For this review, use the dimensioned drawing (mm, ordinates from the lowest corner) and the shaded views. Coordinates: 2 decimals unless noted, no trailing zeros. Loops run counter-clockwise (first coordinate to the right, second up) from the corner with the lowest first, then second, coordinate; pieces in that order, holes last.
1. Take a section at A-A, the plane x = 105. State the section outline as (y, z) points.
2. Take a section at C-C, the plane y = 4.5. State the section outline as (x, z) points.
3. Clearance check with a flat-ended pin moving along its axis: P1, Ø14.5, axis at x = 283, z = 11, coming from the -Y side. State where the tip first meets the part, or that it passes through.
4. To check wall thickness, follow probe 1 along X at (y, z) = (6, 283); probe 2 along X at (y, z) = (5.5, 28); probe 3 along Z at (x, y) = (216, 1.5). State the ranges of each line that lie inside material, in increasing order.
5. Take a section at B-B, the plane z = 220.5. State the section outline as (x, y) points.
6. Take a section at D-D, the plane z = 283. State the section outline as (x, y) points.
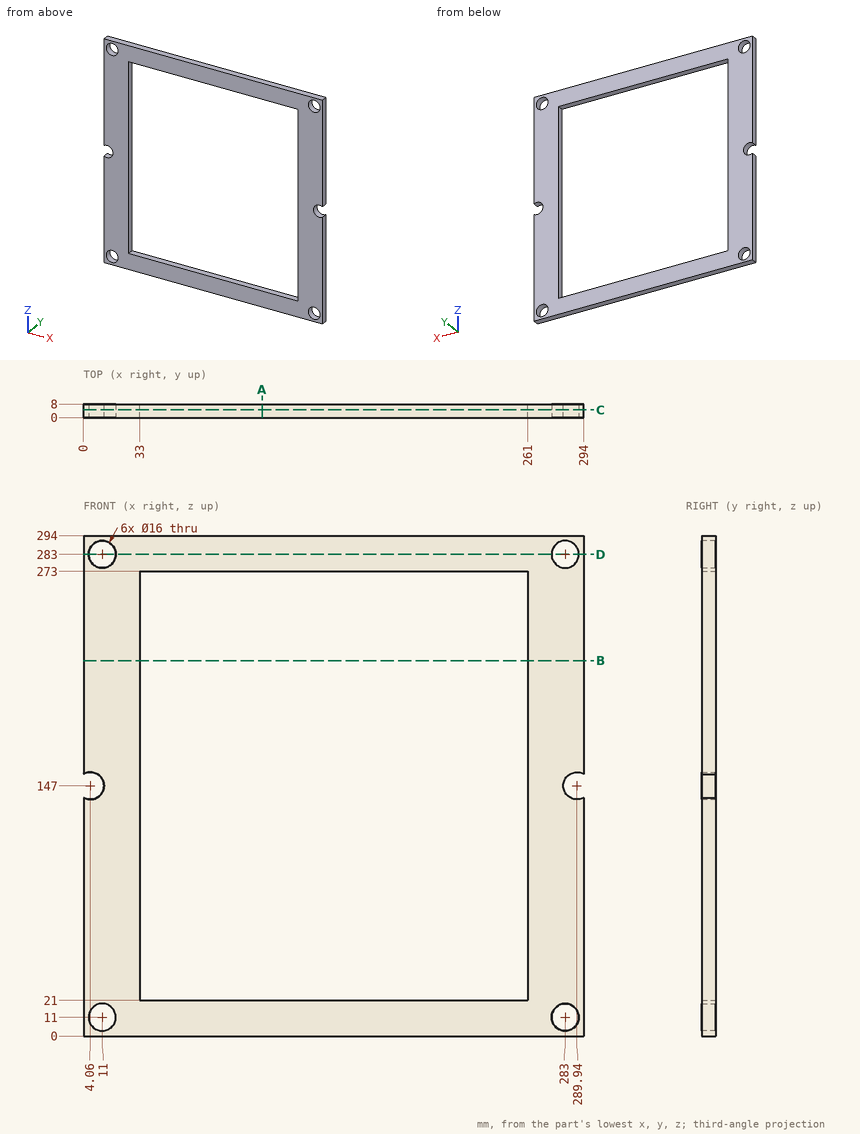
Results list:
1. outline: (0, 0) - (8, 0) - (8, 21) - (0, 21) - close; (0, 273) - (8, 273) - (8, 294) - (0, 294) - close
2. outline: (0, 0) - (294, 0) - (294, 140.11) arc R8 cw (long way) to (294, 153.89) - (294, 294) - (0, 294) - (0, 153.89) arc R8 cw (long way) to (0, 140.11) - close; hole circle Ø16 at (11, 11); hole circle Ø16 at (11, 283); hole (33, 21) - (261, 21) - (261, 273) - (33, 273) - close; hole circle Ø16 at (283, 11); hole circle Ø16 at (283, 283)
3. P1: passes through
4. probe 1: x = 0 to 3, 19 to 275, 291 to 294
4. probe 2: x = 0 to 33, 261 to 294
4. probe 3: z = 0 to 21, 273 to 294
5. outline: (0, 0) - (33, 0) - (33, 8) - (0, 8) - close; (261, 0) - (294, 0) - (294, 8) - (261, 8) - close
6. outline: (0, 0) - (3, 0) - (3, 8) - (0, 8) - close; (19, 0) - (275, 0) - (275, 8) - (19, 8) - close; (291, 0) - (294, 0) - (294, 8) - (291, 8) - close
